Geometry check sheet. Reference: the model listing, model coordinates, mm. A direction names the side the tool comes from. Coordinates: 2 decimals unless noted, no trailing zeros. Write each loop counter-clockwise with the first axis right and the second up, starting at its lowest first coordinate (ties: lowest second). Pieces come first, ordered by that corner, then holes. Notation, with made-up numbers: (66.5, 35.5) -> (96.5, 35.5) arc R8 ccw to (96.5, 39.5) -> close; hole circle Ø9 at (-19.5, 76.25). An arc over 180 degrees is marked (long way). Answer in a Markdown table with one row per item. Add a question column.
Q1. Thickness scan on line 1 (Z direction, x = 3.5, y = 14.5); line 2 (Z direction, x = 17.5, y = 13.25); line 3 (Y direction, x = -9, z = 68). Record the ranges inside material, lowest first.
Q2. Section check A-A, the plane z = 100. Record the boundary of the cut face in (x, y), and give its area (3 significant figures).
Q3. Section check C-C, the plane x = -12. Count the separate pieces of the cut face and the enclosed holes in it, and give its area (3 significant figures).
Q4. Release check for a two-part mould opening along Z. For faces 1 (the face through (7, 0, 16)), 2 (the face through (-3.35, 8.24, 46.13)) record: pulls with the +Z half, pulls with the -Z half, needs draft (parallel to the pull), parting line crosses it, or undercut.
Q5. Section check B-B, the plane z = 132. Record the boundary of the cut face in (x, y).
Q6. Gauge pin test, flat ends, axial feed: P1, Ø5.5, axis at x = 2, z = 79.5, coming from the +Y side; P2, Ø12, axis at x = 2, z = 52.5, coming from the -Y side; P3, Ø1, axis at x = 26, y = 3, coming from the -Z side; P4, Ø3.5, axis at x = 7.53, z = 164.97, coming from the +Y side. Record the tip position at first contact, or that the pin passes through.
Q7. Tool access check on faces 3 (the face through (19.347, 5.728, 31.447)), 4 (the face through (-3.588, 8.374, 101.789)), 5 (the face through (-15.265, 6, 94)). Record the directions out of +Z, -Z, +X, -X, +Y, -Y that give a thin tool (end or side, any length) a straight path to the whole face; none if there is none.
```python
from build123d import *

# Parameters (mm, degrees)
SKETCH1_R           = 2.25
SKETCH1_R_2         = 2.65
SKETCH1_R_3         = 2.15
BOSS_EXTRUDE1_DEPTH = 15
CUT_EXTRUDE2_DEPTH  = 46
SKETCH3_W           = 23.685590182
SKETCH3_H           = 96.44516038
CUT_EXTRUDE4_DEPTH  = 1
SKETCH4_W           = 23.685590182
SKETCH4_H           = 96.44516038
CUT_EXTRUDE5_DEPTH  = 1


with BuildPart() as part:
    # Sketch1 → Boss-Extrude1 (new body)
    with BuildSketch(Plane(origin=(0, 0, 0), x_dir=(1, 0, 0), z_dir=(0, 1, 0))):
        with BuildLine():
            Line((-15.264606027, -1.25325428), (-15.264606027, -189.971404395))
            Line((-15.264606027, -189.971404395), (16.735393973, -189.971404395))
            ThreePointArc((16.735393973, -189.971404395), (22.392248222, -187.628258644), (24.735393973, -181.971404395))
            Line((24.735393973, -181.971404395), (24.735393973, -154.971404395))
            Line((24.735393973, -154.971404395), (8.420984155, -138.656994577))
            Line((8.420984155, -138.656994577), (8.420984155, -42.211834197))
            Line((8.420984155, -42.211834197), (30.584014254, -20.376885374))
            Line((30.584014254, -20.376885374), (30.429434292, 0))
            Line((30.429434292, 0), (20.736580617, 10.028595605))
            Line((20.736580617, 10.028595605), (-3.982756142, 10.028595605))
            Line((-3.982756142, 10.028595605), (-15.264606027, -1.25325428))
        make_face()
        with Locations(Location((-5.264606027, -179.971404395, 0), (0, 0, 270))):
            Circle(SKETCH1_R, mode=Mode.SUBTRACT)
        with Locations(Location((7.525634834, -179.971404395, 0), (0, 0, 270))):
            Circle(SKETCH1_R, mode=Mode.SUBTRACT)
        with Locations(Location((-5.264606027, -164.971404395, 0), (0, 0, 270))):
            Circle(SKETCH1_R, mode=Mode.SUBTRACT)
        with Locations(Location((7.525634834, -164.971404395, 0), (0, 0, 270))):
            Circle(SKETCH1_R, mode=Mode.SUBTRACT)
        with Locations(Location((8.5, -10, 0), (0, 0, 270))):
            Circle(SKETCH1_R_2, mode=Mode.SUBTRACT)
        with Locations(Location((0, 0, 0), (0, 0, 270))):
            Circle(SKETCH1_R_3, mode=Mode.SUBTRACT)
        with Locations(Location((17, 0, 0), (0, 0, 270))):
            Circle(SKETCH1_R_3, mode=Mode.SUBTRACT)
        with Locations(Location((0, -20, 0), (0, 0, 270))):
            Circle(SKETCH1_R_3, mode=Mode.SUBTRACT)
        with Locations(Location((17, -20, 0), (0, 0, 270))):
            Circle(SKETCH1_R_3, mode=Mode.SUBTRACT)
    extrude(amount=BOSS_EXTRUDE1_DEPTH)

    # Sketch2 → Cut-Extrude2 (cut)
    with BuildSketch(Plane.ZY.offset(15.264606027)):
        Polygon((174.971404395, 13.113981192), (174.971404395, 2), (162.971404395, 2), align=None)
        Polygon((149.78200197, 13.113981192), (169.066554165, 13.113981192), (158.686135815, 3.5), align=None)
        Polygon((4.75786812, 3.5), (4.75786812, 13.113981192), (13.66200197, 13.113981192), align=None)
        Polygon((143.88200197, 13.113981192), (152.786135815, 3.5), (143.88200197, 3.5), (134.97786812, 3.5), align=None)
        Polygon((112.80200197, 13.113981192), (121.706135815, 3.5), (112.80200197, 3.5), (103.89786812, 3.5), align=None)
        Polygon((81.72200197, 13.113981192), (90.626135815, 3.5), (81.72200197, 3.5), (72.81786812, 3.5), align=None)
        Polygon((50.64200197, 13.113981192), (59.546135815, 3.5), (50.64200197, 3.5), (41.73786812, 3.5), align=None)
        Polygon((19.56200197, 13.113981192), (28.466135815, 3.5), (19.56200197, 3.5), (10.65786812, 3.5), align=None)
        Polygon((137.986554165, 13.113981192), (127.606135815, 3.5), (118.70200197, 13.113981192), align=None)
        Polygon((106.906554165, 13.113981192), (96.526135815, 3.5), (87.62200197, 13.113981192), align=None)
        Polygon((75.826554165, 13.113981192), (65.446135815, 3.5), (56.54200197, 13.113981192), align=None)
        Polygon((44.746554165, 13.113981192), (34.366135815, 3.5), (25.46200197, 13.113981192), align=None)
    extrude(amount=-CUT_EXTRUDE2_DEPTH, mode=Mode.SUBTRACT)

    # Sketch3 → Cut-Extrude4 (cut)
    with BuildSketch(Plane.XZ):
        with Locations((-3.421810936, 90.434414387)):
            Rectangle(SKETCH3_W, SKETCH3_H)
    extrude(amount=-CUT_EXTRUDE4_DEPTH, mode=Mode.SUBTRACT)

    # Sketch4 → Cut-Extrude5 (cut)
    with BuildSketch(Plane(origin=(0, 15, 0), x_dir=(1, 0, 0), z_dir=(0, 1, 0))):
        with Locations((-3.421810936, -90.434414387)):
            Rectangle(SKETCH4_W, SKETCH4_H)
    extrude(amount=-CUT_EXTRUDE5_DEPTH, mode=Mode.SUBTRACT)


solid = part.part
```
Calculated:
| question | item | result |
|---|---|---|
| 1 | line 1 | z = -10.03 to 42.21, 138.66 to 189.97 |
| 1 | line 2 | z = -10.03 to -2.09, 2.09 to 17.91, 22.09 to 33.27, 147.74 to 189.93 |
| 1 | line 3 | y = 1 to 5.87, 13.11 to 14 |
| 2 | outline | (-15.26, 1) -> (8.42, 1) -> (8.42, 6.72) -> (-15.26, 6.72) -> close; (-15.26, 13.11) -> (8.42, 13.11) -> (8.42, 14) -> (-15.26, 14) -> close |
| 2 | area | 156 mm² |
| 3 | separate pieces | 1 |
| 3 | enclosed holes | 12 |
| 3 | area | 1,690 mm² |
| 4 | face 1 | needs draft |
| 4 | face 2 | undercut |
| 5 | outline | (-15.26, 1) -> (8.42, 1) -> (8.42, 7.57) -> (-15.26, 7.57) -> close; (-15.26, 13.11) -> (8.42, 13.11) -> (8.42, 14) -> (-15.26, 14) -> close |
| 6 | P1 | stops at y = 14 |
| 6 | P2 | stops at y = 1 |
| 6 | P3 | stops at z = -5.1 |
| 6 | P4 | passes through |
| 7 | face 3 | +X, +Y, -Y |
| 7 | face 4 | +X, -X |
| 7 | face 5 | +Z, -Z, -X, +Y, -Y |
